Read the model definition and answer for the solid it produces. Units are mm, in the model's axes. Face numbers are marked on the shaded views. Coordinates: 2 decimals unless noted, no trailing zeros. Loops run counter-clockwise (first coordinate to the right, second up) from the corner with the lowest first, then second, coordinate; pieces in that order, holes last.
Q1. Section D-D (z = 9.75) is taken. Give the vertices of the cut face in (x, y), then the cut area to 3 significant figures.
Q2. Flat-ended cylindrical pins translate along their axes: P1, Ø3, axis at x = 0, z = 13, coming from the +Y side; P2, Ø4, axis at y = 2, z = 7, coming from the +X side; P3, Ø3, axis at x = 1, z = 11, coming from the -Y side; P4, Ø3, axis at y = -1, z = 3.5, coming from the -X side. Find the tip coordinate at first contact, or state that the pin passes through.
Q3. Straight lines are drawn through the part: line 1 (Z direction, x = 4.5, y = -3.5); line 2 (Y direction, x = 0, z = 6); line 3 (Y direction, x = 4.5, z = 8.25). For each, find the intervals that lie inside material, in ascending order.
Q4. The mould has two halves that part along Z. Classify the marked faces 1, 2 and 3: pulls with the +Z half, pulls with the -Z half, needs draft (parallel to the pull), parting line crosses it, or undercut.
Q5. Section B-B (x = 0) is taken. Give the vertices of the cut face in (y, z), then the cut area to 3 significant figures.
Q6. Section A-A (y = 6) is taken. Give the vertices of the cut face in (x, z), then the cut area to 3 significant figures.
from build123d import *

# Parameters (mm, degrees)
F0_R     = 5
F1_DEPTH = 15
F2_R     = 7
F2_R_2   = 2.75
F3_DEPTH = 1
F4_R     = 7
F5_DEPTH = 1


with BuildPart() as f1:
    # F0 (on Top) → F1 (new body)
    with BuildSketch(Plane.XY):
        Circle(F0_R)
    extrude(amount=F1_DEPTH)

    # F2 (on Top) → F3 (join)
    with BuildSketch(Plane.XY):
        Circle(F2_R)
        Circle(F2_R_2, mode=Mode.SUBTRACT)
    extrude(amount=F3_DEPTH)

    # F4 (on face) → F5 (join)
    with BuildSketch(Plane.XY.offset(15)):
        Circle(F4_R)
    extrude(amount=-F5_DEPTH)


solid = f1.part
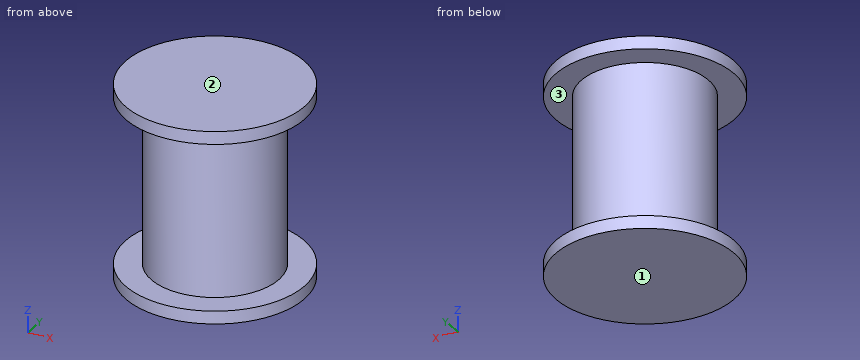
Numbers:
1. outline: circle Ø10 at (0, 0)
1. area: 78.5 mm2
2. P1: stops at y = 7
2. P2: stops at x = 5
2. P3: stops at y = -5
2. P4: stops at x = -5
3. line 1: z = 0 to 1, 14 to 15
3. line 2: y = -5 to 5
3. line 3: y = -2.18 to 2.18
4. face 1: pulls with the -Z half
4. face 2: pulls with the +Z half
4. face 3: undercut
5. outline: (-7, 0) - (7, 0) - (7, 1) - (5, 1) - (5, 14) - (7, 14) - (7, 15) - (-7, 15) - (-7, 14) - (-5, 14) - (-5, 1) - (-7, 1) - close
5. area: 158 mm2
6. outline: (-3.61, 0) - (3.61, 0) - (3.61, 1) - (-3.61, 1) - close; (-3.61, 14) - (3.61, 14) - (3.61, 15) - (-3.61, 15) - close
6. area: 14.4 mm2
